```python
from build123d import *

# Parameters (mm, degrees)
CROQUIS1_W              = 26.4
CROQUIS1_H              = 30.1
SALIENTE_EXTRUIR1_DEPTH = 1.5
CROQUIS3_R              = 1.475
SALIENTE_EXTRUIR3_DEPTH = 26.4


with BuildPart() as part:
    # Croquis1 → Saliente-Extruir1 (new body)
    with BuildSketch(Plane.XY):
        with Locations((14.119367589, -6.959881423)):
            Rectangle(CROQUIS1_W, CROQUIS1_H)
    extrude(amount=SALIENTE_EXTRUIR1_DEPTH)

    # Croquis3 → Saliente-Extruir3 (add)
    with BuildSketch(Plane(origin=(27.319367589, 0, 0), x_dir=(0, 0, -1), z_dir=(1, 0, 0))):
        with BuildLine():
            Line((0, -22.009881423), (-2.400129029, -23.809709392))
            ThreePointArc((-2.400129029, -23.809709392), (-5.88456292, -22.721048598), (-3.75, -19.759612628))
            Line((-3.75, -19.759612628), (-1.5, -19.759612628))
            Line((-1.5, -19.759612628), (0, -22.009881423))
        make_face()
        with Locations((-3.75, -22.009612628)):
            Circle(CROQUIS3_R, mode=Mode.SUBTRACT)
    extrude(amount=-SALIENTE_EXTRUIR3_DEPTH)


solid = part.part
```
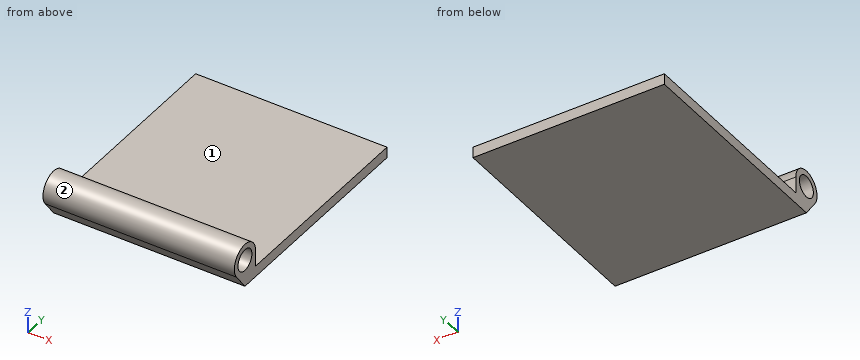
Source: CAD feature listing. Evaluate the final solid. Frame: model axes, mm. Face numbers are marked on the shaded views. A direction names the side the tool comes from. Give positions to 0.01 mm unless a question says otherwise; leave off trailing zeros. Loops run counter-clockwise (first coordinate to the right, second up) from the corner with the lowest first, then second, coordinate; pieces in that order, holes last. Notation, with made-up numbers: (-33.5, 14) - (11.5, 14) arc R17 ccw to (11.5, 29) - close; hole circle Ø3 at (69, 5). An arc over 180 degrees is marked (long way). Use CSV: the item, a comma, the result in double quotes. Start each with the question number.
1. Section B-B (x = 25.5). Output: boundary loops of the cut face in (y, z) (3 decimals), then the cut area to 3 significant figures.
2. Ray query, L1, parallel to Y at x = 12.5, z = 3.75; L2, parallel to Y at x = 8, z = 2.9; L3, parallel to Z at x = 2.25, y = 6.5. Return the intervals inside material, ascending.
3. Section C-C (y = 5). Output: boundary loops of the cut face in (x, z).
4. Pin query (flat end, axial travel): pin 1 (8 mm diameter, centred on x = 15, y = -6.5, fed in from +Z); pin 2 (1 mm diameter, centred on x = 8.5, z = 3, fed in from -Y). Return the tip coordinate at first contact, or that it passes through.
5. Reachability of the marked faces 1 and 2 from +Z, -Z, +X, -X, +Y, -Y: full face, straight path, thin tool, end or side. Return the list, or none.
6. Section A-A (z = 4.85). Output: boundary loops of the cut face in (x, y), then the cut area to 4 significant figures.
Response:
1,outline,"(-23.81, 2.4) - (-22.01, 0) - (8.09, 0) - (8.09, 1.5) - (-19.76, 1.5) - (-19.76, 3.75) arc R2.25 ccw (long way) to start; hole circle Ø2.95 at (-22.01, 3.75)"
1,area,"56.3 mm²"
2,L1,"-24.26 to -23.48, -20.53 to -19.76"
2,L2,"-24.09 to -23.22, -20.8 to -19.76"
2,L3,"0 to 1.5"
3,outline,"(0.92, 0) - (27.32, 0) - (27.32, 1.5) - (0.92, 1.5) - close"
4,pin 1,"z = 1.5"
4,pin 2,"y = -24.25"
5,face 1,"+Z, +X, -X, +Y"
5,face 2,"+X, -X"
6,outline,"(0.92, -23.97) - (27.32, -23.97) - (27.32, -22.99) - (0.92, -22.99) - close; (0.92, -21.03) - (27.32, -21.03) - (27.32, -20.05) - (0.92, -20.05) - close"
6,area,"51.75 mm²"
